```python
from build123d import *

# Parameters (mm, degrees)
SKETCH3_R               = 0.5
SKETCH3_R_2             = 1
CUT_EXTRUDE1_DEPTH      = 5
CUT_EXTRUDE1_DEPTH_BACK = 5


with BuildPart() as part:
    # Sketch1 → Revolve1 (revolve)
    with BuildSketch(Plane.XY):
        Polygon((0, 0), (0, 2.5), (10, 2.5), (10, 3.5), (0, 3.5), (0, 4), (-0.5, 4), (-0.5, 3.5), (-1.5, 2.5), (-3.5, 2.5), (-4.5, 3.5), (-4.5, 4), (-5, 4), (-5, 0), align=None)
    revolve(axis=Axis((0, 0, 0), (-1, 0, 0)))

    # Sketch3 → Cut-Extrude1 (cut, two sides)
    with BuildSketch(Plane.XY) as cut_extrude1_sk:
        with Locations((-2.5, 0)):
            Circle(SKETCH3_R)
        with Locations((5, 0)):
            Circle(SKETCH3_R_2)
    extrude(amount=CUT_EXTRUDE1_DEPTH, mode=Mode.SUBTRACT)
    extrude(cut_extrude1_sk.sketch, amount=-CUT_EXTRUDE1_DEPTH_BACK, mode=Mode.SUBTRACT)


solid = part.part
```
Here's how the part is built. I have some questions about the finished solid (model axes, mm). A direction names the side the tool comes from. Round coordinates to 2 decimals unless told otherwise and drop trailing zeros. Loops run counter-clockwise (first coordinate to the right, second up) from the corner with the lowest first, then second, coordinate; pieces in that order, holes last. Notation, with made-up numbers: (33.25, 71) -> (72.25, 71) arc R12 cw to (72.25, 81) -> close; hole circle Ø2 at (-39, 2). An arc over 180 degrees is marked (long way). Answer as CSV lines item,"result". Start each with the question number.
1. For faces 4 (the face through (4.93, 3.233, 1.341)), 5 (the face through (-5, 0, 0)), 6 (the face through (-2.51, 1.15, 2.22)), which set-ups out of +Z, -Z, +X, -X, +Y, -Y let a thin tool reach every point of the face, with its end or its side?
2. If we mould it in two halves opening along Z, with no side actions, what happens to faces 1 (the face through (-4.754, -0.867, 3.905)), 2 (the face through (0, 0, 0)), 3 (the face through (5, -1, 3))? For each: pulls with the +Z half, pulls with the -Z half, needs draft (parallel to the pull), parting line crosses it, or undercut.
3. Imagine slicing it at A-A on z = 0. Write out the boundary of the cut face in (x, y).
4. I'm going to push flat-ended pins straight in: P1, Ø2.5, axis at y = 0, z = 1, coming from the +X side; P2, Ø2.5, axis at x = 5, y = 0, coming from the +Z side; P3, Ø1.5, axis at x = 2.5, z = 2, coming from the -Y side. Where does each tip first touch, or does it pass through?
5. I need wall thicknesses on probe 1 along X at (y, z) = (0, 0.7); probe 2 along X at (y, z) = (2, 3); probe 3 along X at (y, z) = (0, 3.25). Which ranges of each line are inside material? Lowest first, please. Write a range as from..to.
6. Imagine slicing it at C-C on y = 0. State how many separate pieces and enclosed holes the cut face has, plus the area to 3 significant figures.
7. Imagine slicing it at B-B on x = 5.5. Write out the boundary of the cut face in (y, z), plus the area to 3 significant figures.
Solution:
1,face 4,"+X"
1,face 5,"+Z, -Z, -X, +Y, -Y"
1,face 6,"none"
2,face 1,"parting line crosses it"
2,face 2,"undercut"
2,face 3,"needs draft"
3,outline,"(-5, -4) -> (-4.5, -4) -> (-4.5, -3.5) -> (-3.5, -2.5) -> (-1.5, -2.5) -> (-0.5, -3.5) -> (-0.5, -4) -> (0, -4) -> (0, -3.5) -> (10, -3.5) -> (10, -2.5) -> (0, -2.5) -> (0, 2.5) -> (10, 2.5) -> (10, 3.5) -> (0, 3.5) -> (0, 4) -> (-0.5, 4) -> (-0.5, 3.5) -> (-1.5, 2.5) -> (-3.5, 2.5) -> (-4.5, 3.5) -> (-4.5, 4) -> (-5, 4) -> close; hole circle Ø1 at (-2.5, 0)"
4,P1,"x = 0"
4,P2,"z = 3.5"
4,P3,"y = -3.27"
5,probe 1,"-5..-3, -2..0"
5,probe 2,"-5..-4.5, -0.5..0"
5,probe 3,"-5..-4.25, -0.75..4, 6..10"
6,separate pieces,"4"
6,enclosed holes,"0"
6,area,"41.0 mm²"
7,outline,"(-0.87, -3.39) -> (-0.87, -2.35) arc R2.5 cw to (-0.87, 2.35) -> (-0.87, 3.39) arc R3.5 ccw to start; (0.87, -3.39) arc R3.5 ccw to (0.87, 3.39) -> (0.87, 2.35) arc R2.5 cw to (0.87, -2.35) -> close"
7,area,"15.3 mm²"
